The figure shows three views and two pictorial views of one solid part (mm, origin at its lowest corner). Answer the questions. A direction names the side the tool comes from. Coordinates: 2 decimals unless noted, no trailing zeros. Write each loop counter-clockwise with the first axis right and the second up, starting at its lowest first coordinate (ties: lowest second). Pieces come first, ordered by that corner, then holes. Notation, with made-up numbers: M 69,42.25 L 103,42.25 A26 ccw 103,77.25 Z; hole C 64.5,22 d9. An arc over 180 degrees is marked long. Use CSV: the item, a comma, the result in double quotes.
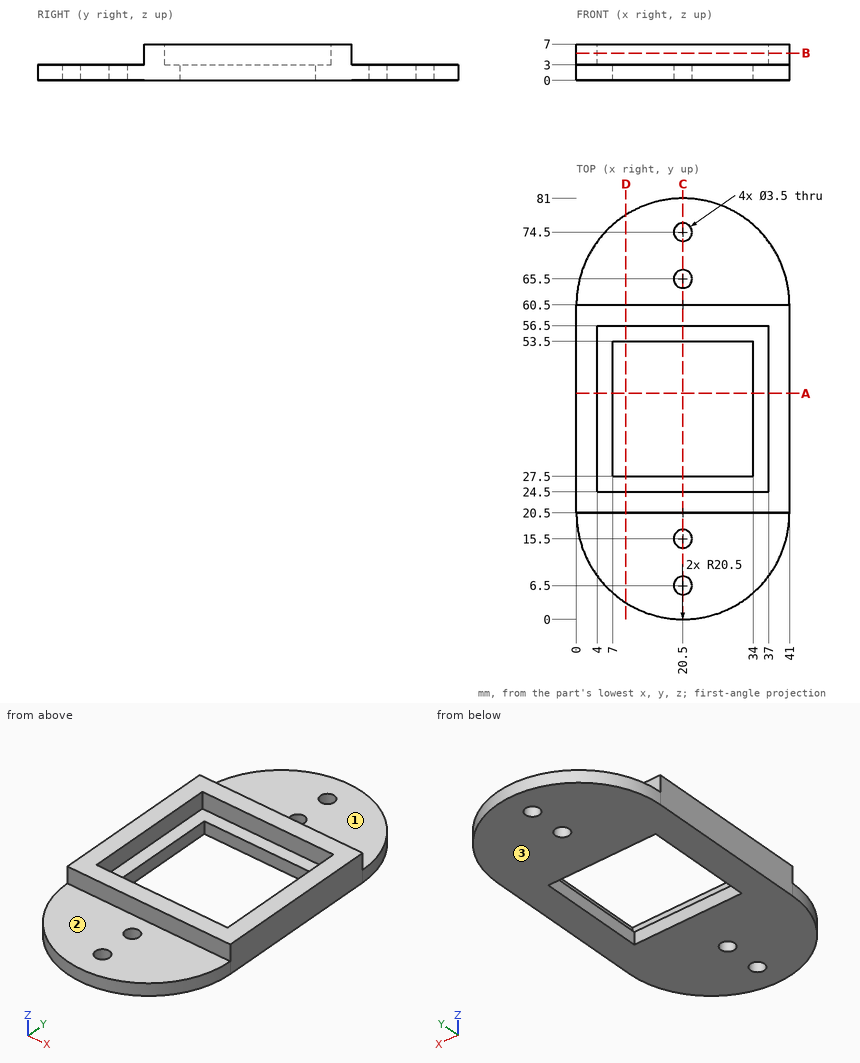
Item 1: Consider probe 1 along Y at (x, z) = (20.5, 1.3); probe 2 along X at (y, z) = (31, 2.75); probe 3 along X at (y, z) = (47, 4.75). Determine where each line is inside the solid, lowest interval first.
Answer:
probe 1,"y = 0 to 4.75, 8.25 to 13.75, 17.25 to 27.5, 53.5 to 63.75, 67.25 to 72.75, 76.25 to 81"
probe 2,"x = 0 to 7, 34 to 41"
probe 3,"x = 0 to 4, 37 to 41"
Item 2: The part is cut by section C-C (x = 20.5). Count the separate pieces of the cut face and the enclosed holes in it, then the cut area to 3 significant figures.
Answer:
separate pieces,"6"
enclosed holes,"0"
area,"155 mm2"
Item 3: The part is cut by section D-D (x = 9.5). Write down the section's boundary in (y, z).
Answer:
outline,"M 3.2,0 L 27.5,0 L 27.5,3 L 24.5,3 L 24.5,7 L 20.5,7 L 20.5,3 L 3.2,3 Z; M 53.5,0 L 77.8,0 L 77.8,3 L 60.5,3 L 60.5,7 L 56.5,7 L 56.5,3 L 53.5,3 Z"
Item 4: A tool of negligible diameter and unlimited length cuts with its end or side. For the marked faces 1, 2 and 3, from which of +Z, -Z, +X, -X, +Y, -Y can it reach the whole face along a straight path? Write none if from no direction.
Answer:
face 1,"+Z, +X, -X, +Y"
face 2,"+Z, +X, -X, -Y"
face 3,"-Z, +X, -X, +Y, -Y"
Item 5: Given pin 1 (1 mm diameter, centred on x = 25, z = 2.5, fed in from +Y); pin 2 (1.2 mm diameter, centred on x = 16, z = 5.5, fed in from -Y); pin 3 (2 mm diameter, centred on x = 20.5, y = 6.5, fed in from -Z); pin 4 (2 mm diameter, centred on x = 21.5, z = 5.5, fed in from +Y), each flat-ended and moving along its own axis, determine where each tip first touches the part or whether it passes through.
Answer:
pin 1,"stops at y = 80.61"
pin 2,"stops at y = 20.5"
pin 3,"passes through"
pin 4,"stops at y = 60.5"
Item 6: The part is cut by section A-A (y = 43.5). Write down the section's boundary in (x, z), then the cut area to 3 significant figures.
Answer:
outline,"M 0,0 L 7,0 L 7,3 L 4,3 L 4,7 L 0,7 Z; M 34,0 L 41,0 L 41,7 L 37,7 L 37,3 L 34,3 Z"
area,"74.0 mm2"
Item 7: The part is cut by section B-B (z = 5.25). Write down the section's boundary in (x, y), then the cut area to 3 significant figures.
Answer:
outline,"M 0,20.5 L 41,20.5 L 41,60.5 L 0,60.5 Z; hole M 4,24.5 L 37,24.5 L 37,56.5 L 4,56.5 Z"
area,"584 mm2"
